```python
from build123d import *

# Parameters (mm, degrees)
SKETCH1_R                 = 25.4
BASE_DEPTH                = 20.6
SKETCH2_R                 = 5.3
BUTTON_DEPTH              = 4.8
F_5_0MM_DOWEL_HOLE1_D     = 5
F_5_0MM_DOWEL_HOLE1_DEPTH = 10.2
F_5_0MM_DOWEL_HOLE1_TIP   = 1.502151548


with BuildPart() as part:
    # Sketch1 → base (new body)
    with BuildSketch(Plane(origin=(0, 0, 0), x_dir=(1, 0, 0), z_dir=(0, 1, 0))):
        Circle(SKETCH1_R)
    extrude(amount=BASE_DEPTH)

    # Sketch2 → button (add)
    with BuildSketch(Plane(origin=(0, 20.6, 0), x_dir=(1, 0, 0), z_dir=(0, 1, 0))):
        Circle(SKETCH2_R)
    extrude(amount=BUTTON_DEPTH)

    # Sketch3 → cable (revolve)
    with BuildSketch(Plane.XY):
        Polygon((-25.075504061, 10.527856927), (-125.419033552, 10.527856927), (-125.419033552, 12.943392514), (-47.075504061, 12.943392514), (-47.075504061, 17.060710463), (-25.075504061, 17.060710463), (-19.522492217, 17.060710463), (-19.522492217, 10.527856927), align=None)
    revolve(axis=Axis((-25.075504061, 10.527856927, 0), (-1, 0, 0)))

    # Ø5.0mm Dowel Hole1
    with Locations(Plane(origin=(-19.771021996, 0, 8.189425453), x_dir=(0, 0, -1), z_dir=(0, -1, 0))):
        with Locations((0, 0), (-11.581596543, 11.581596543), (-11.581596543, 27.960447449), (0, 39.542043992), (16.378850906, 39.542043992), (27.960447449, 27.960447449), (27.960447449, 11.581596543), (16.378850906, 0)):
            Hole(F_5_0MM_DOWEL_HOLE1_D / 2, depth=F_5_0MM_DOWEL_HOLE1_DEPTH)
            with Locations((0, 0, -(F_5_0MM_DOWEL_HOLE1_DEPTH + F_5_0MM_DOWEL_HOLE1_TIP / 2))):  # 118° drill point
                Cone(0, F_5_0MM_DOWEL_HOLE1_D / 2, F_5_0MM_DOWEL_HOLE1_TIP, mode=Mode.SUBTRACT)


solid = part.part
```
Here's how the part is built. I have some questions about the finished solid (model axes, mm). A direction names the side the tool comes from. Coordinates: 2 decimals unless noted, no trailing zeros. Order: outer loops, then holes, each group sorted by start corner. A loop starts at its lowest first (then second) coordinate and runs counter-clockwise, first axis right, second up. Notation, with made-up numbers: M -7.5,69 L 13.5,69 A36 ccw 13.5,105 Z; hole C 86.25,46 d8. An arc over 180 degrees is marked long. Answer as a JSON object with one key per item and string values. Group by question number.
(1) Suppose I cut it at C-C, the plane z = 0. Please give me the cut outline in (x, y) (1 decimal), then the cut area to 3 significant figures.
(2) I need wall thicknesses on probe 1 along Z at (x, y) = (-18, 8.25); probe 2 along Z at (x, y) = (-20, 1.75). Which ranges of each line are inside material? Lowest first, please.
(3) Suppose I cut it at B-B, the plane x = 0. Please give me the cut outline in (y, z).
(4) If we mould it in two halves opening along X, with no side actions, what happens to faces 4 (the face through (24.227, 10.156, -7.629)), 5 (the face through (7.232, 5.171, -17.462)), 6 (the face through (0, 0, 0))? For each: released by +X, released by -X, zero draft, split by the parting line, or undercut.
(5) For pin 1 (12 mm diameter, centred on y = 22, z = 14.5, fed in from +X); pin 2 (6.5 mm diameter, centred on x = -8.19, z = -19.77, fed in from +Y); pin 3 (5 mm diameter, centred on x = -46, z = 6, fed in from +Y), each with a flat end and sliding along its axis, tell me the tip position at first contact or that it passes through.
(6) Suppose I cut it at A-A, the plane y = 2.5. State how many separate pieces and enclosed holes the cut face has, then the cut area to 3 significant figures.
(7) Which directions (+Z, -Z, +X, -X, +Y, -Y) give clear straight access to the entire face, cutting with the end or side of a thin tool? Please do faces 1 (the face through (-9.711, 5.171, 17.787)), 2 (the face through (-36, 5.7, -4.4)), 3 (the face through (0, 20.6, -6)).
(8) Suppose I cut it at D-D, the plane x = -39. Please give me the cut outline in (y, z), then the cut area to 3 significant figures.
Values found:
{
 "1": {"outline": "M -125.4,8.1 L -47.1,8.1 L -47.1,4 L -25.4,4 L -25.4,0 L 25.4,0 L 25.4,20.6 L 5.3,20.6 L 5.3,25.4 L -5.3,25.4 L -5.3,20.6 L -25.4,20.6 L -25.4,17.1 L -47.1,17.1 L -47.1,12.9 L -125.4,12.9 Z", "area": "1,760 mm^2"},
 "2": {"probe 1": "z = -17.92 to -9.95, -6.42 to 6.42, 9.95 to 17.92", "probe 2": "z = -15.66 to -10.68, -5.7 to 5.7, 10.68 to 15.66"},
 "3": {"outline": "M 0,-25.4 L 20.6,-25.4 L 20.6,-5.3 L 25.4,-5.3 L 25.4,5.3 L 20.6,5.3 L 20.6,25.4 L 0,25.4 Z"},
 "4": {"face 4": "split by the parting line", "face 5": "undercut", "face 6": "zero draft"},
 "5": {"pin 1": "stops at x = 23.88", "pin 2": "stops at y = 20.6", "pin 3": "stops at y = 16.04"},
 "6": {"separate pieces": "1", "enclosed holes": "8", "area": "1,870 mm^2"},
 "7": {"face 1": "-Y", "face 2": "-X", "face 3": "+Y"},
 "8": {"outline": "C 10.53,0 d13.07", "area": "134 mm^2"}
}
